Build history of the part. All positions in model axes, mm. Coordinates: 2 decimals unless noted, no trailing zeros. Loops run counter-clockwise (first coordinate to the right, second up) from the corner with the lowest first, then second, coordinate; pieces in that order, holes last.
(1) Slice it at B-B (z = 985). Give the cut face in (x, y).
(2) Slice it at D-D (y = -114). Give the cut face in (x, z).
(3) Wall check: L1, parallel to Y at x = 0.5, z = 268; L2, parallel to Y at x = -7, z = 205; L3, parallel to X at y = -34, z = 887. Give the ranges that are in metal, low to high.
(4) Flat gauge pins, fed straight in: P1, Ø12, axis at x = -12.5, y = 21, coming from the +Z side; P2, Ø8, axis at y = -45.5, z = 727, coming from the +X side; P3, Ø5, axis at x = 18.5, z = 251, coming from the +Y side; P4, Ø8, axis at x = 7.5, z = 518.5, coming from the -Y side. Where does each tip first touch, or does it go through?
(5) Slice it at A-A (y = 0). Give the cut face in (x, z), and give its area (3 significant figures).
(6) Slice it at C-C (y = 65.5). Give the cut face in (x, z), and give its area (3 significant figures).
from build123d import *

# Parameters (mm, degrees)
F0_R          = 50
F0_R_2        = 30
F1_DEPTH      = 1000
F3_R          = 14.7596932235
F4_DEPTH      = 100
F4_DEPTH_BACK = 7
F6_R          = 15
F7_DEPTH      = 100
F7_DEPTH_BACK = 7


with BuildPart() as f1:
    # F0 (on Top) → F1 (new body)
    with BuildSketch(Plane.XY):
        Circle(F0_R)
        Circle(F0_R_2, mode=Mode.SUBTRACT)
    extrude(amount=F1_DEPTH)

    # F3 (on offset) → F4 (join, two sides)
    with BuildSketch(Plane.XZ.offset(50)) as f4_sk:
        with Locations((0, 15)):
            Circle(F3_R)
    extrude(amount=F4_DEPTH)
    extrude(f4_sk.sketch, amount=-F4_DEPTH_BACK)

    # F6 (on offset) → F7 (join, two sides)
    with BuildSketch(Plane.XZ.offset(-50)) as f7_sk:
        with Locations((0, 985)):
            Circle(F6_R)
    extrude(amount=-F7_DEPTH)
    extrude(f7_sk.sketch, amount=F7_DEPTH_BACK)


solid = f1.part
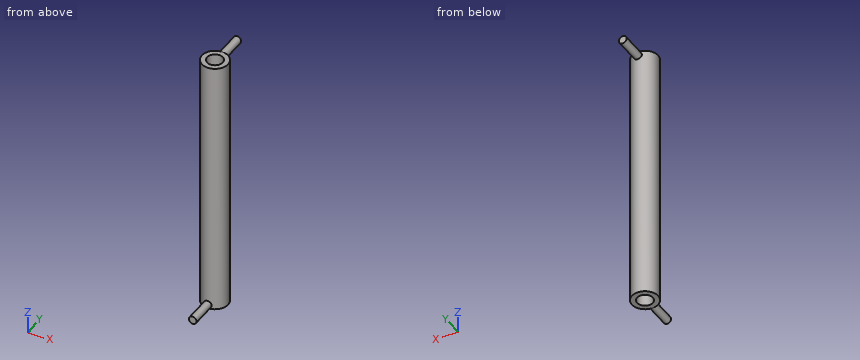
Response values:
1. outline: (-15, 47.7) arc R50 ccw (long way) to (15, 47.7) - (15, 150) - (-15, 150) - close; hole circle Ø60 at (0, 0)
2. outline: circle Ø29.52 at (0, 15)
3. L1: y = -50 to -30, 30 to 50
3. L2: y = -49.51 to -29.17, 29.17 to 49.51
3. L3: x = -36.66 to 36.66
4. P1: stops at z = 1000
4. P2: stops at x = 27.89
4. P3: stops at y = 47.37
4. P4: stops at y = -49.88
5. outline: (-50, 0) - (-30, 0) - (-30, 1000) - (-50, 1000) - close; (30, 0) - (50, 0) - (50, 1000) - (30, 1000) - close
5. area: 40,000 mm2
6. outline: circle Ø30 at (0, 985)
6. area: 707 mm2
